```python
from build123d import *


with BuildPart() as part:
    # Sketch1 → Base-Revolve (revolve)
    with BuildSketch(Plane.XY, mode=Mode.PRIVATE) as base_revolve_sk:
        Polygon((0, 0), (0, 2.437306696), (2.1, 3), (29.2, 3), (30, 2.785640646), (30, 2.15), (29, 2.15), (28.711324865, 1.65), (20, 1.65), (19.008579979, 0), align=None)
    revolve(base_revolve_sk.sketch.rotate(Axis((-10, 0, 0), (1, 0, 0)), 90), axis=Axis((-10, 0, 0), (1, 0, 0)))

    # Sketch2 → TypeA (revolve, cut)
    with BuildSketch(Plane.XY, mode=Mode.PRIVATE) as typea_sk:
        with BuildLine():
            Line((0.590443768, 2.595515627), (0.590443768, 8))
            Line((0.590443768, 8), (-5, 8))
            Line((-5, 8), (-5, 0))
            Line((-5, 0), (0, 0))
            ThreePointArc((0, 0), (0.149472785, 1.33091371), (0.590443768, 2.595515627))
        make_face()
    revolve(typea_sk.sketch.rotate(Axis((0, 0, 0), (1, 0, 0)), 180), axis=Axis((0, 0, 0), (1, 0, 0)), mode=Mode.SUBTRACT)


solid = part.part
```
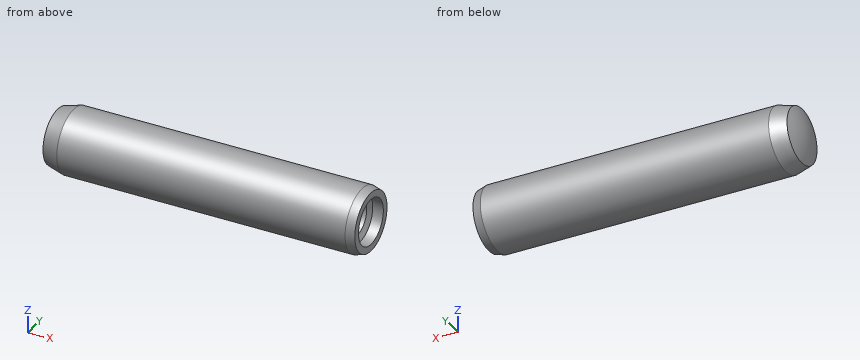
Check sheet for the modelled part. Datum: model origin and axes. Units: mm. Round coordinates to 2 decimals unless told otherwise and drop trailing zeros. Write each loop counter-clockwise with the first axis right and the second up, starting at its lowest first coordinate (ties: lowest second). Pieces come first, ordered by that corner, then holes. Notation, with made-up numbers: (-12.5, -14.5) -> (35.5, -14.5) arc R16 cw to (35.5, -8.5) -> close; hole circle Ø1 at (-12.5, 50.5). An arc over 180 degrees is marked (long way). One line per question, with ' | ' between items. Start each with the question number.
1. Sectioned sample at A-A, the plane x = 22.25. Record the cut outline in (y, z).
2. Scan lines: line 1 along Y through (x, z) = (24.25, 0); line 2 along Z through (x, y) = (9.25, -1.5); line 3 along Y through (x, z) = (29.5, 0). Record each from-to range of solid material in increasing order. Write a range as from..to.
3. Depth check by flat-ended pin: pin 1 (1 mm diameter, centred on x = 24, z = 1, fed in from +Y). Enter the tip coordinate at first touch or a pass-through.
4. Sectioned sample at B-B, the plane x = 12. Record the cut outline in (y, z), then the cut area to 3 significant figures.
Taken from the geometry:
1) outline: circle Ø6 at (0, 0); hole circle Ø3.3 at (0, 0)
2) line 1: y = -3..-1.65, 1.65..3 | line 2: z = -2.6..2.6 | line 3: y = -2.92..-2.15, 2.15..2.92
3) pin 1: stops at y = 2.96
4) outline: circle Ø6 at (0, 0) | area: 28.3 mm^2
